```python
from build123d import *

# Parameters (mm, degrees)
F1_DEPTH  = 50
F3_DEPTH  = 88
F4_R      = 25
F5_DEPTH  = 115
F7_DEPTH  = 50
F8_W      = 16
F8_H      = 48.0000468988
F9_DEPTH  = 88
F11_DEPTH = 27.7
F12_R     = 8.5
F13_DEPTH = 57.3
F15_DEPTH = 109.8


with BuildPart() as f1:
    # F0 (on Front) → F1 (new body)
    with BuildSketch(Plane.XZ):
        Polygon((-74.9091474319, 0), (0, 0), (0, 88), (-75, 88), align=None)
    extrude(amount=F1_DEPTH)

    # F2 (on face) → F3 (join)
    with BuildSketch(Plane.XY.offset(88)):
        with BuildLine():
            Line((0, -50), (-75, -50))
            ThreePointArc((-75, -50), (-37.5, -87.5), (0, -50))
        make_face()
    extrude(amount=-F3_DEPTH)

    # F4 (on face) → F5 (cut)
    with BuildSketch(Plane.XY.offset(88)):
        with Locations((-37.5, -50)):
            Circle(F4_R)
    extrude(amount=-F5_DEPTH, mode=Mode.SUBTRACT)

    # F6 (on face) → F7 (join)
    with BuildSketch(Plane(origin=(0, 0, 0), x_dir=(-1, 0, 0), z_dir=(0, 1, 0))):
        Polygon((74.9504440318, 39.9999786824), (74.9091474319, 0), (162.9091005331, -0.0908525197), (162.950397133, 39.9091261627), align=None)
    extrude(amount=-F7_DEPTH)

    # F8 (on face) → F9 (join)
    with BuildSketch(Plane(origin=(-74.9090675877, 0, -0.077337286), x_dir=(0, -1, 0), z_dir=(-0.9999994671, 0, -0.001032415))):
        with Locations((8, 64.0773607766)):
            Rectangle(F8_W, F8_H)
    extrude(amount=F9_DEPTH)

    # F10 (on face) → F11 (cut)
    with BuildSketch(Plane.XZ.offset(16)):
        Polygon((-162.9999531012, 87.9091474803), (-162.950397133, 39.9091261627), (-75, 88), align=None)
    extrude(amount=-F11_DEPTH, mode=Mode.SUBTRACT)

    # F12 (on face) → F13 (cut)
    with BuildSketch(Plane(origin=(-0.0413764441, 0, 40.0773159683), x_dir=(0.9999994671, 0, 0.001032415), z_dir=(-0.001032415, 0, 0.9999994671))):
        with Locations((-118.9338855071, -33)):
            Circle(F12_R)
    extrude(amount=-F13_DEPTH, mode=Mode.SUBTRACT)

    # F14 (on face) → F15 (cut)
    with BuildSketch(Plane.XZ.offset(50)):
        with BuildLine():
            Line((-137.9184055916, 8.9349530588), (-118.9184157175, 8.9545689437))
            Line((-118.9184157175, 8.9545689437), (-99.9297824083, 8.9349530588))
            ThreePointArc((-99.9297824083, 8.9349530588), (-88.9086009647, 19.9447551389), (-99.9297824083, 30.954557219))
            Line((-99.9297824083, 30.954557219), (-118.9411288474, 30.954557219))
            Line((-118.9411288474, 30.954557219), (-137.9184055916, 30.954557219))
            ThreePointArc((-137.9184055916, 30.954557219), (-148.9282076717, 19.9447551389), (-137.9184055916, 8.9349530588))
        make_face()
    extrude(amount=-F15_DEPTH, mode=Mode.SUBTRACT)


solid = f1.part
```
The model under review builds one solid part; all positions refer to its coordinate system, in mm. A direction names the side the tool comes from. Round coordinates to 2 decimals unless told otherwise and drop trailing zeros. Order: outer loops, then holes, each group sorted by start corner. A loop starts at its lowest first (then second) coordinate and runs counter-clockwise, first axis right, second up. Notation, with made-up numbers: (32.25, 89.25) -> (54.25, 89.25) arc R32 cw to (54.25, 120.25) -> close; hole circle Ø7 at (40.5, 74). An arc over 180 degrees is marked (long way). Use a Markdown table: item, result.
Q1. We need section B-B on y = -45.5. Write out the cut boundary in (x, z).
Values:
| item | result |
|---|---|
| outline | (-162.95, 39.91) -> (-162.91, -0.09) -> (-74.91, 0) -> (-62.09, 0) -> (-62.09, 88) -> (-75, 88) -> (-74.95, 40) -> close; (-12.91, 0) -> (0, 0) -> (0, 88) -> (-12.91, 88) -> close; hole (-137.92, 8.93) -> (-118.92, 8.95) -> (-99.93, 8.93) arc R11.01 ccw to (-99.93, 30.95) -> (-137.92, 30.95) arc R11.01 ccw to start |
Q2. Clearance check with flat-ended pins moving along their axes: P1, Ø20, axis at x = -107.5, z = 27.5, coming from the -Y side; P2, Ø2, axis at x = -103.5, z = 42.5, coming from the -Y side; P3, Ø3, axis at y = -47.5, z = 34, coming from the -X side. State where each tip first meets the part, or that it passes through.
Values:
| item | result |
|---|---|
| P1 | stops at y = -50 |
| P2 | stops at y = -16 |
| P3 | stops at x = -162.95 |
Q3. Tool access review of faces 1 (the flat face through (-118, -50, 34)), 2 (the flat face through (-109, -16, 58)), 3 (the flat face through (-114, -25, 30.955)): name each direction out of +Z, -Z, +X, -X, +Y, -Y from which nothing blocks a thin tool from reaching the whole face with its end or side.
Values:
| item | result |
|---|---|
| face 1 | +Z, -Z, -X, -Y |
| face 2 | +Z, -X, -Y |
| face 3 | +Y, -Y |
Q4. For line 1 (Y direction, x = -37.5, z = 25.5); line 2 (Z direction, x = -54, y = -81); line 3 (X direction, y = -20, z = 51.5), list the stretches that pass through material, from the lowest coordinate up.
Values:
| item | result |
|---|---|
| line 1 | y = -87.5 to -75, -25 to 0 |
| line 2 | z = 0 to 88 |
| line 3 | x = -74.96 to 0 |
Q5. We need section A-A on x = -37.5. Write out the cut boundary in (y, z).
Values:
| item | result |
|---|---|
| outline | (-87.5, 0) -> (-75, 0) -> (-75, 88) -> (-87.5, 88) -> close; (-25, 0) -> (0, 0) -> (0, 88) -> (-25, 88) -> close |
Q6. Mouldability with a two-part tool opening along Y and no side actions: class faces 4 (the flat face through (-62, 0, 43)), 5 (the cylindrical face through (-88.91, -25.35, 19.7)), 6 (the cylindrical face through (-125.72, -38.17, 35.51)) as +Y half, -Y half, draft (parallel to the pull), parting line (faces both ways), or undercut.
Values:
| item | result |
|---|---|
| face 4 | +Y half |
| face 5 | draft |
| face 6 | undercut |
Q7. We need section D-D on y = -70.5. Write out the cut boundary in (x, z).
Values:
| item | result |
|---|---|
| outline | (-68.9, 0) -> (-51.81, 0) -> (-51.81, 88) -> (-68.9, 88) -> close; (-23.19, 0) -> (-6.1, 0) -> (-6.1, 88) -> (-23.19, 88) -> close |
